from build123d import *

# Parameters (mm, degrees)
F0_W     = 38.1
F0_H     = 25.4
F1_DEPTH = 31.75
F2_W     = 38.1
F2_H     = 15.875
F3_DEPTH = 12.7
F5_DEPTH = 25.4
F7_DEPTH = 25.4


with BuildPart() as f1:
    # F0 (on Top) → F1 (new body)
    with BuildSketch(Plane.XY):
        with Locations((19.05, 12.7)):
            Rectangle(F0_W, F0_H)
    extrude(amount=F1_DEPTH)

    # F2 (on face) → F3 (cut)
    with BuildSketch(Plane.XZ):
        with Locations((19.05, 23.8125)):
            Rectangle(F2_W, F2_H)
    extrude(amount=-F3_DEPTH, mode=Mode.SUBTRACT)

    # F4 (on face) → F5 (cut)
    with BuildSketch(Plane.XZ.offset(-12.7)):
        Polygon((38.1, 15.875), (38.1, 31.75), (25.4, 31.75), align=None)
    extrude(amount=-F5_DEPTH, mode=Mode.SUBTRACT)

    # F6 (on face) → F7 (cut)
    with BuildSketch(Plane(origin=(0, 0, 0), x_dir=(1, 0, 0), z_dir=(0, 0, -1))):
        Polygon((38.1, -10.627423), (38.1, 0), (25.4, 0), align=None)
    extrude(amount=-F7_DEPTH, mode=Mode.SUBTRACT)


solid = f1.part
Work out the finished part from the listing and answer in its coordinate system (mm). A direction names the side the tool comes from. Coordinates: 2 decimals unless noted, no trailing zeros. Write each loop counter-clockwise with the first axis right and the second up, starting at its lowest first coordinate (ties: lowest second). Pieces come first, ordered by that corner, then holes. Notation, with made-up numbers: M 24.5,66 L 31.5,66 A18 ccw 31.5,78 Z; hole C -4.5,71.25 d1. An arc over 180 degrees is marked long. Answer as CSV lines item,"result". Start each with the question number.
Item 1: Section A-A on z = 6 is taken. Write down the section's boundary in (x, y), and give its area (3 significant figures).
Item 2: A tool of negligible diameter and unlimited length cuts with its end or side. For faces 1 (the face through (15, 12.7, 24)), 2 (the face through (19, 13, 0)), from which of +Z, -Z, +X, -X, +Y, -Y can it reach the whole face along a straight path? Write none if from no direction.
Item 3: Section C-C on y = 16 is taken. Write down the section's boundary in (x, z) (3 decimals), and give its area (3 significant figures).
Item 4: Flat-ended cylindrical pins translate along their axes: P1, Ø14, axis at x = 21, y = 4, coming from the +Z side (3 decimals); P2, Ø5, axis at x = 18.5, z = 27.5, coming from the -Y side; P3, Ø1.5, axis at y = 5.5, z = 9, coming from the +X side. Find the tip coordinate at first contact, or state that the pin passes through.
Item 5: Consider L1, parallel to Z at x = 24, y = 4.75 (3 decimals); L2, parallel to Y at x = 14.5, z = 19; L3, parallel to X at y = 19.75, z = 27.5. Determine where each line is inside the solid, lowest interval first.
Item 6: Section B-B on x = 13 is taken. Write down the section's boundary in (y, z) (3 decimals).
Item 7: Section D-D on z = 29 is taken. Write down the section's boundary in (x, y), and give its area (3 significant figures).
Checks:
1,outline,"M 0,0 L 25.4,0 L 38.1,10.63 L 38.1,25.4 L 0,25.4 Z"
1,area,"900 mm²"
2,face 1,"+Z, +X, -X, -Y"
2,face 2,"-Z, +X, -X, +Y, -Y"
3,outline,"M 0,0 L 38.1,0 L 38.1,15.875 L 25.4,31.75 L 0,31.75 Z"
3,area,"1,110 mm²"
4,P1,"stops at z = 15.875"
4,P2,"stops at y = 12.7"
4,P3,"stops at x = 32.87"
5,L1,"z = 0 to 15.875"
5,L2,"y = 12.7 to 25.4"
5,L3,"x = 0 to 28.8"
6,outline,"M 0,0 L 25.4,0 L 25.4,31.75 L 12.7,31.75 L 12.7,15.875 L 0,15.875 Z"
7,outline,"M 0,12.7 L 27.6,12.7 L 27.6,25.4 L 0,25.4 Z"
7,area,"351 mm²"
